from build123d import *

# Parameters (mm, degrees)
BOSS_EXTRUDE1_DEPTH = 1.6002
SKETCH2_W           = 20.32
SKETCH2_H           = 41.275
CUT_EXTRUDE5_DEPTH  = 2.6002
SKETCH3_W           = 50.8
SKETCH3_H           = 50.8
CUT_EXTRUDE6_DEPTH  = 2.54


with BuildPart() as part:
    # Sketch1 → Boss-Extrude1 (new body)
    with BuildSketch(Plane.XY):
        Polygon((0, 0), (50.8, 0), (50.8, 76.2), (400.05, 76.2), (400.05, -38.1), (-400.05, -38.1), (-400.05, 76.2), (0, 76.2), align=None)
    extrude(amount=BOSS_EXTRUDE1_DEPTH)

    # Sketch2 → Cut-Extrude5 (cut, through all)
    with BuildSketch(Plane.XY):
        with Locations((-73.66, 20.6375)):
            Rectangle(SKETCH2_W, SKETCH2_H)
        with Locations((111.76, 20.6375)):
            Rectangle(SKETCH2_W, SKETCH2_H)
    extrude(amount=CUT_EXTRUDE5_DEPTH, mode=Mode.SUBTRACT)

    # Sketch3 → Cut-Extrude6 (cut)
    with BuildSketch(Plane(origin=(0, 0, 0), x_dir=(-1, 0, 0), z_dir=(0, 0, -1))):
        with Locations((25.4, 25.4)):
            Rectangle(SKETCH3_W, SKETCH3_H)
    extrude(amount=-CUT_EXTRUDE6_DEPTH, mode=Mode.SUBTRACT)


solid = part.part
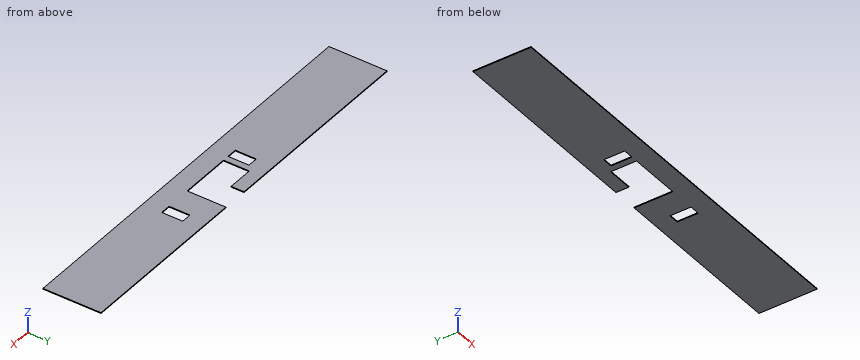
The listing builds one solid part. Answer for the finished solid, in the listing's coordinates (mm). Coordinates: 2 decimals unless noted, no trailing zeros. Write each loop counter-clockwise with the first axis right and the second up, starting at its lowest first coordinate (ties: lowest second). Pieces come first, ordered by that corner, then holes. Notation, with made-up numbers: M 84.25,47 L 109.25,47 A37 ccw 109.25,86 Z; hole C -33.5,1.5 d11. An arc over 180 degrees is marked long. Put each result on its own line as item: value. Start each with the question number.
1. A cutting plane is placed at A-A on y = 27. Write down the section's boundary in (x, z).
2. A cutting plane is placed at C-C on y = 58. Write down the section's boundary in (x, z).
3. A flat-ended cylindrical pin translates along its axis: P1, Ø0.8, axis at x = 23.5, z = 1, coming from the +Y side. Find the tip coordinate at first contact, or state that the pin passes through.
4. A cutting plane is placed at B-B on z = 0.35. Write down the section's boundary in (x, y) (3 decimals).
5. Consider line 1 (X direction, y = 15, z = 0.25); line 2 (Y direction, x = -10.5, z = 1.45); line 3 (X direction, y = 66, z = 0.85). Determine where each line is inside the solid, lowest interval first. Write a range as from..to.
Resolved:
1. outline: M -400.05,0 L -83.82,0 L -83.82,1.6 L -400.05,1.6 Z; M -63.5,0 L -50.8,0 L -50.8,1.6 L -63.5,1.6 Z; M 50.8,0 L 101.6,0 L 101.6,1.6 L 50.8,1.6 Z; M 121.92,0 L 400.05,0 L 400.05,1.6 L 121.92,1.6 Z
2. outline: M -400.05,0 L 0,0 L 0,1.6 L -400.05,1.6 Z; M 50.8,0 L 400.05,0 L 400.05,1.6 L 50.8,1.6 Z
3. P1: stops at y = 0
4. outline: M -400.05,-38.1 L 400.05,-38.1 L 400.05,76.2 L 50.8,76.2 L 50.8,0 L -50.8,0 L -50.8,50.8 L 0,50.8 L 0,76.2 L -400.05,76.2 Z; hole M -83.82,0 L -63.5,0 L -63.5,41.275 L -83.82,41.275 Z; hole M 101.6,0 L 121.92,0 L 121.92,41.275 L 101.6,41.275 Z
5. line 1: x = -400.05..-83.82, -63.5..-50.8, 50.8..101.6, 121.92..400.05
5. line 2: y = -38.1..0, 50.8..76.2
5. line 3: x = -400.05..0, 50.8..400.05
